Could you check a few things on this model? Use its own coordinates, in mm. A direction names the side the tool comes from. Round coordinates to 2 decimals unless told otherwise and drop trailing zeros. Order: outer loops, then holes, each group sorted by start corner. A loop starts at its lowest first (then second) coordinate and runs counter-clockwise, first axis right, second up. Notation, with made-up numbers: (6, 15.25) - (29, 15.25) arc R13 cw to (29, 29.25) - close; hole circle Ø3 at (48.5, 80.25). An arc over 180 degrees is marked (long way). Return JSON: item names as keys, results as strings. Group by question number.
from build123d import *

# Parameters (mm, degrees)
SKETCH_1_R          = 9
SKETCH_1_R_2        = 8
EXTRUDE_1_DEPTH     = 75
EXTRUDE_2_DEPTH     = 10
EXTRUDE_START       = 12
EXTRUDE_3_DEPTH     = 12
SKETCH_4_R          = 5
EXTRUDE_4_DEPTH     = 8
SKETCH_5_R          = 2.5
CUT_EXTRUDE_1_DEPTH = 38
SKETCH_6_R          = 2
SKETCH_6_R_2        = 1.980516498
CUT_EXTRUDE_3_DEPTH = 3


with BuildPart() as part:
    # 草图1 → 凸台-拉伸1 (new body)
    with BuildSketch(Plane.XY):
        Circle(SKETCH_1_R)
        Circle(SKETCH_1_R_2, mode=Mode.SUBTRACT)
    extrude(amount=EXTRUDE_1_DEPTH)

    # 草图2 → 凸台-拉伸2 (add)
    with BuildSketch(Plane.XY.offset(75)):
        with BuildLine():
            Line((-5, -9), (5, -9))
            ThreePointArc((5, -9), (7.828427125, -7.828427125), (9, -5))
            Line((9, -5), (9, 5))
            ThreePointArc((9, 5), (7.828427125, 7.828427125), (5, 9))
            Line((5, 9), (-5, 9))
            ThreePointArc((-5, 9), (-7.828427125, 7.828427125), (-9, 5))
            Line((-9, 5), (-9, -5))
            ThreePointArc((-9, -5), (-7.828427125, -7.828427125), (-5, -9))
        make_face()
    extrude(amount=EXTRUDE_2_DEPTH)

    # 草图3 → 凸台-拉伸3 (add)
    with BuildSketch(Plane(origin=(0, 0, 0), x_dir=(-1, 0, 0), z_dir=(0, 0, -1)).offset(EXTRUDE_START)):
        with BuildLine():
            Line((-5, -9), (5, -9))
            ThreePointArc((5, -9), (7.828427125, -7.828427125), (9, -5))
            Line((9, -5), (9, 5))
            ThreePointArc((9, 5), (7.828427125, 7.828427125), (5, 9))
            Line((5, 9), (-5, 9))
            ThreePointArc((-5, 9), (-7.828427125, 7.828427125), (-9, 5))
            Line((-9, 5), (-9, -5))
            ThreePointArc((-9, -5), (-7.828427125, -7.828427125), (-5, -9))
        make_face()
    extrude(amount=-EXTRUDE_3_DEPTH)

    # 草图4 → 凸台-拉伸4 (add)
    with BuildSketch(Plane(origin=(0, 0, -12), x_dir=(-1, 0, 0), z_dir=(0, 0, -1))):
        Circle(SKETCH_4_R)
    extrude(amount=EXTRUDE_4_DEPTH)

    # 草图5 → 切除-拉伸1 (cut)
    with BuildSketch(Plane(origin=(0, 0, -20), x_dir=(-1, 0, 0), z_dir=(0, 0, -1))):
        Circle(SKETCH_5_R)
    extrude(amount=-CUT_EXTRUDE_1_DEPTH, mode=Mode.SUBTRACT)

    # 草图6 → 切除-拉伸3 (cut)
    with BuildSketch(Plane.ZY.offset(9)):
        with Locations((-4, 0)):
            Circle(SKETCH_6_R)
        with Locations((79, 0)):
            Circle(SKETCH_6_R_2)
    extrude(amount=-CUT_EXTRUDE_3_DEPTH, mode=Mode.SUBTRACT)


solid = part.part
1) If I drill on line 1 along Z through (x, y) = (-2, 4.25); line 2 along Z through (x, y) = (6.75, -8); line 3 along Y through (x, z) = (0, -6), over which ranges is the centre line in solid material (lowest first)? Write a range as from..to.
2) We'd pull the mould along Z, two halves only. Please class faces 5 (the flat face through (4, 4, -12)), 6 (the cylindrical face through (-7.797, -7.859, -6.084)), 7 (the flat face through (-7, 7, 75)): +Z half, -Z half, draft (parallel to the pull), parting line (faces both ways), or undercut.
3) I want a section at C-C, the plane z = 79. List the corners of the cut face in (x, y) for me, plus the area to 3 significant figures.
4) I want a section at B-B, the plane y = -3.75. List the corners of the cut face in (x, z) for me.
5) I want a section at D-D, the plane x = 4. List the corners of the cut face in (y, z) for me.
6) Will these pins go through, and if not, where does the flat tip stop? pin 1 (8 mm diameter, centred on y = -3.5, z = 47, fed in from +X); pin 2 (4 mm diameter, centred on x = 0, y = 0, fed in from -Z); pin 3 (2.5 mm diameter, centred on y = 0, z = -4, fed in from -X); pin 4 (4.5 mm diameter, centred on x = 4.5, y = -6.5, fed in from -Z).
7) For faces 1 (the cylindrical face through (1.08, -4.88, -15.94)), 2 (the flat face through (-7, -7, 75)), 3 (the flat face through (7, 7, 0)), 4 (the cylindrical face through (-1.172, 8.923, 36.975)), which set-ups out of +Z, -Z, +X, -X, +Y, -Y let a thin tool reach every point of the face, with its end or its side?
8) I want a section at A-A, the plane z = -7. List the corners of the cut face in (x, y) for me, plus the area to 3 significant figures.
Outcome:
{
 "1": {"line 1": "-20..0, 75..85", "line 2": "-12..0, 75..85", "line 3": "-9..-2.5, 2.5..9"},
 "2": {"face 5": "-Z half", "face 6": "draft", "face 7": "undercut"},
 "3": {"outline": "(-9, -5) arc R4 ccw to (-5, -9) - (5, -9) arc R4 ccw to (9, -5) - (9, 5) arc R4 ccw to (5, 9) - (-5, 9) arc R4 ccw to (-9, 5) - (-9, 1.98) - (-6, 1.98) - (-6, -1.98) - (-9, -1.98) - close", "area": "298 mm^2"},
 "4": {"outline": "(-9, -12) - (-3.31, -12) - (-3.31, -20) - (3.31, -20) - (3.31, -12) - (9, -12) - (9, 0) - (8.18, 0) - (8.18, 75) - (9, 75) - (9, 85) - (-9, 85) - (-9, 75) - (-8.18, 75) - (-8.18, 0) - (-9, 0) - close; hole (-7.07, 0) - (7.07, 0) - (7.07, 75) - (-7.07, 75) - close"},
 "5": {"outline": "(-9, -12) - (-3, -12) - (-3, -20) - (3, -20) - (3, -12) - (9, -12) - (9, 0) - (8.06, 0) - (8.06, 75) - (9, 75) - (9, 85) - (-9, 85) - (-9, 75) - (-8.06, 75) - (-8.06, 0) - (-9, 0) - close; hole (-6.93, 0) - (6.93, 0) - (6.93, 75) - (-6.93, 75) - close"},
 "6": {"pin 1": "x = 9", "pin 2": "z = 75", "pin 3": "x = -6", "pin 4": "z = -12"},
 "7": {"face 1": "-Z", "face 2": "-X, -Y", "face 3": "+X, +Y", "face 4": "none"},
 "8": {"outline": "(-9, -5) arc R4 ccw to (-5, -9) - (5, -9) arc R4 ccw to (9, -5) - (9, 5) arc R4 ccw to (5, 9) - (-5, 9) arc R4 ccw to (-9, 5) - close; hole circle Ø5 at (0, 0)", "area": "291 mm^2"}
}
